from build123d import *

# Parameters (mm, degrees)
F0_W     = 25.4
F0_H     = 127
F1_DEPTH = 25.4
F2_T     = -1.5875
F3_W     = 25.4
F3_H     = 127
F4_DEPTH = 6.35
F5_R     = 6.35
F6_DEPTH = 31.751


with BuildPart() as f1:
    # F0 (on Top) → F1 (new body)
    with BuildSketch(Plane.XY):
        Rectangle(F0_W, F0_H)
    extrude(amount=F1_DEPTH)

    # F2
    f2_openings = [f1.faces().sort_by_distance(p)[0] for p in [
        (0, -63.5, 12.7),
    ]]
    offset(amount=F2_T, openings=f2_openings)

    # F3 (on face) → F4 (join)
    with BuildSketch(Plane.XY.offset(25.4)):
        Rectangle(F3_W, F3_H)
        Polygon((-12.7, -63.5), (-12.7, 63.5), (-88.9, -38.1), (-88.9, -63.5), align=None)
    extrude(amount=F4_DEPTH)

    # F5 (on face) → F6 (cut, through all)
    with BuildSketch(Plane(origin=(0, 0, 0), x_dir=(1, 0, 0), z_dir=(0, 0, -1))):
        with Locations((0, -44.897698)):
            Circle(F5_R)
    extrude(amount=-F6_DEPTH, mode=Mode.SUBTRACT)


solid = f1.part
Input: part model. Units: mm. Frame: model coordinates. A direction names the side the tool comes from. Give positions to 0.01 mm unless a question says otherwise; leave off trailing zeros. Order: outer loops, then holes, each group sorted by start corner. A loop starts at its lowest first (then second) coordinate and runs counter-clockwise, first axis right, second up. Notation, with made-up numbers: (64, 47.5) - (121, 47.5) arc R20 ccw to (121, 64.5) - close; hole circle Ø11 at (-7, 26). An arc over 180 degrees is marked (long way). Answer as a JSON object with one key per item and string values. Group by question number.
Q1. Cut plane A-A, the plane y = 15.5. Output: boundary loops of the cut face in (x, z), then the cut area to 3 significant figures.
Q2. Cut plane D-D, the plane y = -42. Output: boundary loops of the cut face in (x, z).
Q3. Mould query, pull axis X, two halves, no side actions, for faces 1 (the face through (0, 1, 0)), 2 (the face through (-88.9, -51, 29)), 3 (the face through (0, 61.912, 13)). Classes: pulls with the +X half, pulls with the -X half, needs draft (parallel to the pull), parting line crosses it, or undercut.
Q4. First-contact query: pin 1 Ø4 at (x, y) = (-31, -37.5) entering from -Z; pin 2 Ø8 at (x, z) = (-43, 26) entering from +Y; pin 3 Ø11 at (y, z) = (0, 8) entering from -X. Flat tips, straight axial feed; report the tip coordinate or a pass-through.
Q5. Line query: probe 1 along X at (y, z) = (-19, 9); probe 2 along Z at (x, y) = (8, -55); probe 3 along Y at (x, z) = (0, 0.4). Output: solid intervals per line, ascending.
Q6. Cut plane B-B, the plane x = 0. Output: boundary loops of the cut face in (y, z).
Q7. Set-up query: faces 4 (the face through (11.112, -2, 13)), 5 (the face through (-43, -13, 25.4)), 6 (the face through (12.7, -1, 16)). Return all of +Z, -Z, +X, -X, +Y, -Y with unobstructed straight access to the full face (end or side cutting, diameter ignored); none if empty.
Q8. Cut plane C-C, the plane z = 8. Output: boundary loops of the cut face in (x, y).
Results:
{
 "1": {"outline": "(-48.7, 25.4) - (-12.7, 25.4) - (-12.7, 0) - (12.7, 0) - (12.7, 31.75) - (-48.7, 31.75) - close; hole (-11.11, 1.59) - (11.11, 1.59) - (11.11, 23.81) - (-11.11, 23.81) - close", "area": "541 mm^2"},
 "2": {"outline": "(-88.9, 25.4) - (-12.7, 25.4) - (-12.7, 0) - (12.7, 0) - (12.7, 31.75) - (-88.9, 31.75) - close; hole (-11.11, 1.59) - (11.11, 1.59) - (11.11, 23.81) - (-11.11, 23.81) - close"},
 "3": {"face 1": "needs draft", "face 2": "pulls with the -X half", "face 3": "undercut"},
 "4": {"pin 1": "z = 25.4", "pin 2": "y = 28.43", "pin 3": "x = -12.7"},
 "5": {"probe 1": "-12.7 to -11.11, 11.11 to 12.7", "probe 2": "0 to 1.59, 23.81 to 31.75", "probe 3": "-63.5 to 38.55, 51.25 to 63.5"},
 "6": {"outline": "(-63.5, 0) - (38.55, 0) - (38.55, 1.59) - (-63.5, 1.59) - close; (-63.5, 23.81) - (38.55, 23.81) - (38.55, 31.75) - (-63.5, 31.75) - close; (51.25, 0) - (63.5, 0) - (63.5, 31.75) - (51.25, 31.75) - (51.25, 23.81) - (61.91, 23.81) - (61.91, 1.59) - (51.25, 1.59) - close"},
 "7": {"face 4": "-Y", "face 5": "-Z, -X, +Y, -Y", "face 6": "+Z, -Z, +X, +Y, -Y"},
 "8": {"outline": "(-12.7, -63.5) - (-11.11, -63.5) - (-11.11, 61.91) - (11.11, 61.91) - (11.11, -63.5) - (12.7, -63.5) - (12.7, 63.5) - (-12.7, 63.5) - close"}
}
